The model under review builds one solid part; all positions refer to its coordinate system, in mm. A direction names the side the tool comes from. Give positions to 0.01 mm unless a question says otherwise; leave off trailing zeros. Loops run counter-clockwise (first coordinate to the right, second up) from the corner with the lowest first, then second, coordinate; pieces in that order, holes last. Notation, with made-up numbers: (47.25, -12.5) - (106.25, -12.5) arc R25 cw to (106.25, 4.5) - close; hole circle Ø8 at (-4, 25). An arc over 180 degrees is marked (long way). Answer as a JSON object with one key per item and string values.
from build123d import *

# Parameters (mm, degrees)
BOSS_EXTRUDE1_DEPTH      = 3
BOSS_EXTRUDE2_DEPTH      = 3
SKETCH3_W                = 100
SKETCH3_H                = 4
BOSS_EXTRUDE3_DEPTH      = 20
CUT_EXTRUDE1_DEPTH       = 106
BOSS_EXTRUDE4_DEPTH      = 58
SKETCH6_W                = 100
SKETCH6_H                = 39.623225513
BOSS_EXTRUDE5_DEPTH      = 3
BOSS_EXTRUDE6_REACH      = 101.805
SKETCH7_W                = 4
SKETCH7_H                = 22.901045637
SKETCH10_R               = 2
CUT_EXTRUDE3_DEPTH       = 10
BOSS_EXTRUDE8_REACH      = 89.321
SKETCH12_R               = 2
CUT_EXTRUDE4_DEPTH       = 88.321245983
SKETCH13_W               = 90
SKETCH13_H               = 7
CUT_EXTRUDE5_DEPTH       = 3
CUT_EXTRUDE6_START       = -21
SKETCH15_R               = 4
SKETCH15_R_2             = 2
CUT_EXTRUDE6_DEPTH       = 21
BOSS_EXTRUDE9_DEPTH      = 1
BOSS_EXTRUDE9_DEPTH_BACK = 3
SKETCH16_R               = 4
SKETCH16_R_2             = 2
SKETCH17_W               = 83
SKETCH17_H               = 48.5
SKETCH17_W_2             = 77
SKETCH17_H_2             = 42.5
BOSS_EXTRUDE10_DEPTH     = 5


with BuildPart() as part:
    # Sketch1 → Boss-Extrude1 (new body)
    with BuildSketch(Plane(origin=(0, 0, 0), x_dir=(1, 0, 0), z_dir=(0, 1, 0))):
        Polygon((-50, 45), (50, 45), (50, -45), (45, -45), (45, 40), (-45, 40), (-45, -45), (-50, -45), align=None)
    extrude(amount=BOSS_EXTRUDE1_DEPTH)

    # Sketch2 → Boss-Extrude2 (add)
    with BuildSketch(Plane.XY.offset(45)):
        Polygon((-50, 3), (-50, 30), (50, 30), (50, 3), (45, 3), (45, 23), (-45, 23), (-45, 3), align=None)
    extrude(amount=-BOSS_EXTRUDE2_DEPTH)

    # Sketch3 → Boss-Extrude3 (add)
    with BuildSketch(Plane.XY.offset(45)):
        with Locations((0, 28)):
            Rectangle(SKETCH3_W, SKETCH3_H)
    extrude(amount=BOSS_EXTRUDE3_DEPTH)

    # Sketch4 → Cut-Extrude1 (cut)
    with BuildSketch(Plane(origin=(50, 0, 0), x_dir=(0, 0, -1), z_dir=(1, 0, 0))):
        Polygon((-65, 26), (-65, 30), (-63, 30), align=None)
    extrude(amount=-CUT_EXTRUDE1_DEPTH, mode=Mode.SUBTRACT)

    # Sketch5 → Boss-Extrude4 (add)
    with BuildSketch(Plane(origin=(0, 0, 42), x_dir=(-1, 0, 0), z_dir=(0, 0, -1))):
        Polygon((-50, 3), (-46, 3), (-46, 27), (46, 27), (46, 3), (50, 3), (50, 30), (-50, 30), align=None)
    extrude(amount=BOSS_EXTRUDE4_DEPTH)

    # Sketch6 → Boss-Extrude5 (add)
    with BuildSketch(Plane(origin=(0, 24.049681529, -22.391082803), x_dir=(-1, 0, 0), z_dir=(0, -0.7318939744313501, 0.6814185279188426))):
        with Locations((0, 11.07936051)):
            Rectangle(SKETCH6_W, SKETCH6_H)
    extrude(amount=BOSS_EXTRUDE5_DEPTH)

    # Sketch7 → Boss-Extrude6 (add, up to next)
    with BuildSketch(Plane(origin=(0, 0, -16), x_dir=(-1, 0, 0), z_dir=(0, 0, -1)), mode=Mode.PRIVATE) as boss_extrude6_sk1:
        with Locations((-48, 14.450522819)):
            Rectangle(SKETCH7_W, SKETCH7_H)
    boss_extrude6_tool1 = extrude(boss_extrude6_sk1.sketch, amount=BOSS_EXTRUDE6_REACH, mode=Mode.PRIVATE) - part.part
    # Sketch7 → Boss-Extrude6 (add, up to next)
    with BuildSketch(Plane(origin=(0, 0, -16), x_dir=(-1, 0, 0), z_dir=(0, 0, -1)), mode=Mode.PRIVATE) as boss_extrude6_sk2:
        with Locations((48, 14.450522819)):
            Rectangle(SKETCH7_W, SKETCH7_H)
    boss_extrude6_tool2 = extrude(boss_extrude6_sk2.sketch, amount=BOSS_EXTRUDE6_REACH, mode=Mode.PRIVATE) - part.part
    add(boss_extrude6_tool1.solids().sort_by_distance((48, 14.450523, -16))[0])
    add(boss_extrude6_tool2.solids().sort_by_distance((-48, 14.450523, -16))[0])

    # Sketch10 → Cut-Extrude3 (cut)
    with BuildSketch(Plane(origin=(0, 30, 0), x_dir=(1, 0, 0), z_dir=(0, 1, 0))):
        with Locations(Location((40, -55, 0), (0, 0, 180))):
            Circle(SKETCH10_R)
        with Locations(Location((-40, -55, 0), (0, 0, 180))):
            Circle(SKETCH10_R)
    extrude(amount=-CUT_EXTRUDE3_DEPTH, mode=Mode.SUBTRACT)

    # Boss-Extrude8: up to this plane
    boss_extrude8_end = Plane(origin=(0, 21.853999605, -20.346827219), z_dir=(0, -0.7318939744313501, 0.6814185279188426))
    # Sketch11 → Boss-Extrude8 (add, up to the surface)
    with BuildSketch(Plane.XZ, mode=Mode.PRIVATE) as boss_extrude8_sk1:
        with BuildLine():
            Line((-40, -33), (-48.829023615, -33))
            Line((-48.829023615, -33), (-48.829023615, -41))
            Line((-48.829023615, -41), (-40, -41))
            ThreePointArc((-40, -41), (-36, -37), (-40, -33))
        make_face()
    boss_extrude8_tool1 = split(extrude(boss_extrude8_sk1.sketch, amount=-BOSS_EXTRUDE8_REACH, mode=Mode.PRIVATE), bisect_by=boss_extrude8_end, keep=Keep.BOTH, mode=Mode.PRIVATE)
    add(boss_extrude8_tool1.solids().sort_by_distance((-42.810423, 0, -37))[0])
    # Sketch11 → Boss-Extrude8 (add, up to the surface)
    with BuildSketch(Plane.XZ, mode=Mode.PRIVATE) as boss_extrude8_sk2:
        with BuildLine():
            Line((40, -33), (48.614584002, -33))
            Line((48.614584002, -33), (48.614584002, -41))
            Line((48.614584002, -41), (40, -41))
            ThreePointArc((40, -41), (36, -37), (40, -33))
        make_face()
    boss_extrude8_tool2 = split(extrude(boss_extrude8_sk2.sketch, amount=-BOSS_EXTRUDE8_REACH, mode=Mode.PRIVATE), bisect_by=boss_extrude8_end, keep=Keep.BOTH, mode=Mode.PRIVATE)
    add(boss_extrude8_tool2.solids().sort_by_distance((42.702596, 0, -37))[0])

    # Sketch12 → Cut-Extrude4 (cut, through all)
    with BuildSketch(Plane.XZ):
        with Locations(Location((-40, -37, 0), (0, 0, 270))):
            Circle(SKETCH12_R)
        with Locations(Location((40, -37, 0), (0, 0, 270))):
            Circle(SKETCH12_R)
    extrude(amount=-CUT_EXTRUDE4_DEPTH, mode=Mode.SUBTRACT)

    # Sketch13 → Cut-Extrude5 (cut)
    with BuildSketch(Plane.XZ):
        with Locations((0, -36.5)):
            Rectangle(SKETCH13_W, SKETCH13_H)
    extrude(amount=-CUT_EXTRUDE5_DEPTH, mode=Mode.SUBTRACT)

    # Sketch15 → Cut-Extrude6 (cut)
    # profile 1 of 2: a face of its own
    with BuildSketch(Plane(origin=(0, 30, 0), x_dir=(1, 0, 0), z_dir=(0, 1, 0)).offset(CUT_EXTRUDE6_START)):
        with Locations((-40, 37)):
            Circle(SKETCH15_R)
        with Locations(Location((-40, 37, 0), (0, 0, 90))):
            Circle(SKETCH15_R_2, mode=Mode.SUBTRACT)
    # profile 2 of 2: a face of its own
    with BuildSketch(Plane(origin=(0, 30, 0), x_dir=(1, 0, 0), z_dir=(0, 1, 0)).offset(CUT_EXTRUDE6_START)):
        with Locations((40, 37)):
            Circle(SKETCH15_R)
        with Locations(Location((40, 37, 0), (0, 0, 90))):
            Circle(SKETCH15_R_2, mode=Mode.SUBTRACT)
    extrude(amount=CUT_EXTRUDE6_DEPTH, mode=Mode.SUBTRACT)

    # Sketch16 → Boss-Extrude9 (add, two sides: drawn at the far end of the back side and taken through both)
    # profile 1 of 2: a face of its own
    with BuildSketch(Plane(origin=(0, 9, 0), x_dir=(1, 0, 0), z_dir=(0, 1, 0)).offset(-BOSS_EXTRUDE9_DEPTH_BACK)):
        with Locations((-40, 37)):
            Circle(SKETCH16_R)
        with Locations(Location((-40, 37, 0), (0, 0, 90))):
            Circle(SKETCH16_R_2, mode=Mode.SUBTRACT)
    # profile 2 of 2: a face of its own
    with BuildSketch(Plane(origin=(0, 9, 0), x_dir=(1, 0, 0), z_dir=(0, 1, 0)).offset(-BOSS_EXTRUDE9_DEPTH_BACK)):
        with Locations((40, 37)):
            Circle(SKETCH16_R)
        with Locations(Location((40, 37, 0), (0, 0, 90))):
            Circle(SKETCH16_R_2, mode=Mode.SUBTRACT)
    extrude(amount=BOSS_EXTRUDE9_DEPTH + BOSS_EXTRUDE9_DEPTH_BACK)

    # Sketch17 → Boss-Extrude10 (add)
    with BuildSketch(Plane.XZ.offset(-27)):
        with Locations((0, 9.534179837)):
            Rectangle(SKETCH17_W, SKETCH17_H)
        with Locations((0, 9.534179837)):
            Rectangle(SKETCH17_W_2, SKETCH17_H_2, mode=Mode.SUBTRACT)
    extrude(amount=BOSS_EXTRUDE10_DEPTH)


solid = part.part
Q1. For faces 5 (the face through (41.5, 25, 9)), 6 (the face through (-1, 26, 55)), 7 (the face through (-46, 15, 5)), 8 (the face through (-42, 3, -36)), list the 3-axis set-ups (+Z, -Z, +X, -X, +Y, -Y) from which the entire face can be reached by the end or side of a thin tool; tool diameter is ignored.
Results:
{"face 5": "-Y", "face 6": "+Z, +X, -X, -Y", "face 7": "none", "face 8": "+Z, -Y"}
Q2. Consider section D-D, the plane z = -6. State the section outline as (x, y) points, plus the area to 3 significant figures.
Results:
{"outline": "(-50, 0) - (-45, 0) - (-45, 3) - (-46, 3) - (-46, 27) - (-41.5, 27) - (-41.5, 22) - (-38.5, 22) - (-38.5, 27) - (38.5, 27) - (38.5, 22) - (41.5, 22) - (41.5, 27) - (46, 27) - (46, 3) - (45, 3) - (45, 0) - (50, 0) - (50, 30) - (-50, 30) - close", "area": "552 mm^2"}
Q3. The part is to be moulded in two halves that separate along Z. For faces 1 (the face through (45, 1, 9)), 2 (the face through (-42, 6, -37)), 3 (the face through (0.7, 16.311, -30.703)), 4 (the face through (-1, 25, 33.784)), say which applies: +Z half, -Z half, draft (parallel to the pull), parting line (faces both ways), or undercut.
Results:
{"face 1": "draft", "face 2": "undercut", "face 3": "-Z half", "face 4": "undercut"}
Q4. Consider section A-A, the plane z = 55. State the section outline as (x, y) points.
Results:
{"outline": "(-50, 26) - (-42, 26) - (-42, 30) - (-50, 30) - close; (-38, 26) - (38, 26) - (38, 30) - (-38, 30) - close; (42, 26) - (50, 26) - (50, 30) - (42, 30) - close"}
Q5. Consider section B-B, the plane z = 32. State the section outline as (x, y) points.
Results:
{"outline": "(-50, 0) - (-45, 0) - (-45, 3) - (-46, 3) - (-46, 27) - (-41.5, 27) - (-41.5, 22) - (41.5, 22) - (41.5, 27) - (46, 27) - (46, 3) - (45, 3) - (45, 0) - (50, 0) - (50, 30) - (-50, 30) - close"}
Q6. Clearance check with flat-ended pins moving along their axes: pin 1 Ø1.5 at (x, y) = (10.5, 25.5) entering from -Z; pin 2 Ø12 at (x, y) = (-18, 20.5) entering from -Z; pin 3 Ø12 at (x, z) = (-38.5, 41.5) entering from -Y. State where each tip first meets the part, or that it passes through.
Results:
{"pin 1": "stops at z = -21.64", "pin 2": "stops at z = -32.65", "pin 3": "stops at y = 23"}
Q7. Consider section C-C, the plane x = -31.5. State the section outline as (y, z) points.
Results:
{"outline": "(0, -45) - (3, -45) - (30, -16) - (30, 63) - (26, 65) - (26, 45) - (23, 45) - (23, 42) - (27, 42) - (27, 33.78) - (22, 33.78) - (22, 30.78) - (27, 30.78) - (27, -11.72) - (22, -11.72) - (22, -14.72) - (27, -14.72) - (27, -14.82) - (3, -40.6) - (3, -40) - (0, -40) - close"}
Q8. To check wall thickness, follow probe 1 along X at (y, z) = (22.5, 5); probe 2 along X at (y, z) = (5, -37); probe 3 along X at (y, z) = (12, 14). State the ranges of each line that lie inside material, in increasing order. Write a range as [from, to].
Results:
{"probe 1": "x = [-50, -46], [-41.5, -38.5], [38.5, 41.5], [46, 50]", "probe 2": "x = [-50, -42], [-38, -36], [36, 38], [42, 50]", "probe 3": "x = [-50, -46], [46, 50]"}
